from build123d import *

# Parameters (mm, degrees)
F0_W     = 368
F0_H     = 368
F1_DEPTH = 16
F3_D     = 50
F3_DEPTH = 16
F3_TIP   = 15.0215154757
F2_R     = 50
F4_DEPTH = 3
F7_R     = 25
F8_DEPTH = 600
F9_D     = 3
F9_DEPTH = 3
F9_TIP   = 0.9012909285


# Not quite as in the source:
# - the program builds the solid bodies; features that only make, move or delete a surface that nothing else refers to are left out


with BuildPart() as f1:
    # F0 (on Top) → F1 (new body)
    with BuildSketch(Plane.XY):
        Rectangle(F0_W, F0_H)
    extrude(amount=F1_DEPTH)

    # F3
    with Locations(Plane.XY.offset(16)):
        with Locations((-134, -134)):
            Hole(F3_D / 2, depth=F3_DEPTH)
            with Locations((0, 0, -(F3_DEPTH + F3_TIP / 2))):  # 118° drill point
                Cone(0, F3_D / 2, F3_TIP, mode=Mode.SUBTRACT)

    # F2 (on face) → F4 (join)
    with BuildSketch(Plane.XY.offset(16)):
        with Locations((-134, -134)):
            Circle(F2_R)
    extrude(amount=F4_DEPTH)

    # F7 (on face) → F8 (join)
    with BuildSketch(Plane.XY.offset(19)):
        with Locations((-134, -134)):
            Circle(F7_R)
    extrude(amount=F8_DEPTH)

    # F9 (one way)
    with BuildSketch(Plane(origin=(0, 0, 16), x_dir=(1, 0, 0), z_dir=(0, 0, -1))):
        with Locations((-134, 96), (-171.9844305378, 135.0876749154), (-96.0155694622, 135.0876749154), (-134, 172)):
            Circle(F9_D / 2)
    extrude(amount=-F9_DEPTH, mode=Mode.SUBTRACT)
    with Locations(Plane(origin=(0, 0, 16), x_dir=(1, 0, 0), z_dir=(0, 0, -1))):
        with Locations((-134, 96), (-171.9844305378, 135.0876749154), (-96.0155694622, 135.0876749154), (-134, 172)):
            with Locations((0, 0, -(F9_DEPTH + F9_TIP / 2))):  # 118° drill point
                Cone(0, F9_D / 2, F9_TIP, mode=Mode.SUBTRACT)


solid = f1.part
Check sheet for the modelled part. Datum: model origin and axes. Units: mm. A direction names the side the tool comes from. Round coordinates to 2 decimals unless told otherwise and drop trailing zeros. Loops run counter-clockwise (first coordinate to the right, second up) from the corner with the lowest first, then second, coordinate; pieces in that order, holes last.
1. Sectioned sample at C-C on x = 133. Record the boundary of the cut face in (y, z), and give its area (3 significant figures).
2. Set-up check for faces 1 (the flat face through (-134, -134, 16)), 2 (the flat face through (-174, -172, 16)), 3 (the cylindrical face through (-170.852, -100.208, 17.479)): record each of +Z, -Z, +X, -X, +Y, -Y from which the full face is reachable in a straight line by a thin tool's end or side.
3. Scan lines: probe 1 along Y at (x, z) = (-134, 16.85); probe 2 along Z at (x, y) = (-74.5, 24.5); probe 3 along Y at (x, z) = (-134, 11). Record each from-to range of solid material in increasing order.
4. Gauge pin test, flat ends, axial feed: pin 1 Ø1.5 at (x, y) = (-172, -134.5) entering from +Z; pin 2 Ø5 at (x, y) = (-171.98, -135.09) entering from +Z; pin 3 Ø8 at (x, z) = (-117.5, 266) entering from +Y. Record the tip position at first contact, or that the pin passes through.
5. Sectioned sample at A-A on y = -148. Record the boundary of the cut face in (x, z).
6. Sectioned sample at B-B on z = 384. Record the boundary of the cut face in (x, y).
Recorded:
1. outline: (-184, 0) - (184, 0) - (184, 16) - (-184, 16) - close
1. area: 5,890 mm2
2. face 1: -Z
2. face 2: +Z, -X, -Y
2. face 3: +Z
3. probe 1: y = -184 to -173.5, -170.5 to -97.5, -94.5 to -84
3. probe 2: z = 0 to 16
3. probe 3: y = -184 to -159, -109 to 184
4. pin 1: stops at z = 16
4. pin 2: stops at z = 19
4. pin 3: stops at y = -112.35
5. outline: (-184, 0) - (-154.71, 0) - (-154.71, 16) - (-113.29, 16) - (-113.29, 0) - (184, 0) - (184, 16) - (-86, 16) - (-86, 19) - (-113.29, 19) - (-113.29, 619) - (-154.71, 619) - (-154.71, 19) - (-182, 19) - (-182, 16) - (-184, 16) - close
6. outline: circle Ø50 at (-134, -134)
